from build123d import *

# Parameters (mm, degrees)
F0_W      = 50
F0_H      = 70
F1_DEPTH  = 67
F3_DEPTH  = 1.5
F4_W      = 29
F4_H      = 3.3
F5_DEPTH  = 67.001
F7_R      = 20
F8_DEPTH  = 1.5
F10_R     = 20
F11_DEPTH = 1.5
F12_R     = 3.15
F13_DEPTH = 12.5


with BuildPart() as f1:
    # F0 (on Front) → F1 (new body)
    with BuildSketch(Plane.XZ):
        with Locations((-25, 35)):
            Rectangle(F0_W, F0_H)
    extrude(amount=F1_DEPTH)

    # F2 (on face) → F3 (cut)
    with BuildSketch(Plane.YZ):
        Polygon((-67, 70), (-67, 65.2), (-38.1895705521, 35), (-33.5, 39.915755627), (-62.2, 70), align=None)
        Polygon((-33.5, 39.915755627), (-38.1895705521, 35), (-33.5, 30.084244373), (-28.8104294479, 35), align=None)
        Polygon((-67, 4.8), (-67, 0), (-62.2, 0), (-33.5, 30.084244373), (-38.1895705521, 35), align=None)
        Polygon((-4.8, 70), (-33.5, 39.915755627), (-28.8104294479, 35), (0, 65.2), (0, 70), align=None)
        Polygon((-33.5, 30.084244373), (-4.8, 0), (0, 0), (0, 4.8), (-28.8104294479, 35), align=None)
    extrude(amount=-F3_DEPTH, mode=Mode.SUBTRACT)

    # F4 (on face) → F5 (cut, through all)
    with BuildSketch(Plane(origin=(0, 0, 0), x_dir=(-1, 0, 0), z_dir=(0, 1, 0))):
        with Locations((35.5, 55.85)):
            Rectangle(F4_W, F4_H)
        with BuildLine():
            ThreePointArc((46, 27), (45.3525906995, 31.9175618569), (43.4544826719, 36.5))
            ThreePointArc((43.4544826719, 36.5), (8, 27), (43.4544826719, 17.5))
            ThreePointArc((43.4544826719, 17.5), (45.3525906995, 22.0824381431), (46, 27))
        make_face()
        with BuildLine():
            Line((50, 17.5), (50, 36.5))
            Line((50, 36.5), (43.4544826719, 36.5))
            ThreePointArc((43.4544826719, 36.5), (45.3525906995, 31.9175618569), (46, 27))
            ThreePointArc((46, 27), (45.3525906995, 22.0824381431), (43.4544826719, 17.5))
            Line((43.4544826719, 17.5), (50, 17.5))
        make_face()
    extrude(amount=-F5_DEPTH, mode=Mode.SUBTRACT)

    # F7 (on offset) → F8 (cut)
    with BuildSketch(Plane(origin=(0, -12.5, 0), x_dir=(-1, 0, 0), z_dir=(0, 1, 0))):
        with Locations((27, 27)):
            Circle(F7_R)
    extrude(amount=-F8_DEPTH, mode=Mode.SUBTRACT)

    # F10 (on offset) → F11 (cut)
    with BuildSketch(Plane(origin=(0, -56, 0), x_dir=(-1, 0, 0), z_dir=(0, 1, 0))):
        with Locations((27, 27)):
            Circle(F10_R)
    extrude(amount=-F11_DEPTH, mode=Mode.SUBTRACT)

    # F12 (on face) → F13 (cut, through all)
    with BuildSketch(Plane.XY.offset(70)):
        with Locations((-41.7, -33.5)):
            Circle(F12_R)
    extrude(amount=-F13_DEPTH, mode=Mode.SUBTRACT)


solid = f1.part
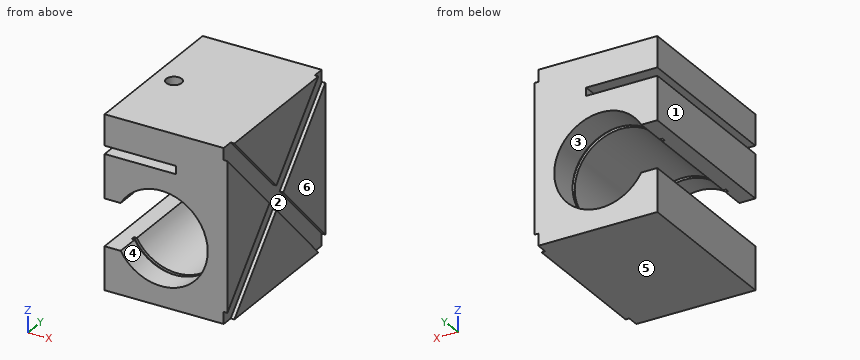
The listing builds one solid part. Answer for the finished solid, in the listing's coordinates (mm). Face numbers are marked on the shaded views. A direction names the side the tool comes from. Give positions to 0.01 mm unless a question says otherwise; leave off trailing zeros. Loops run counter-clockwise (first coordinate to the right, second up) from the corner with the lowest first, then second, coordinate; pieces in that order, holes last. Notation, with made-up numbers: (63, 88.5) - (121, 88.5) arc R23 ccw to (121, 105.5) - close; hole circle Ø11 at (-11.5, 28). An arc over 180 degrees is marked (long way). Write each question's results on one line, items separated by ' | '.
1. Consider probe 1 along Z at (x, y) = (-44.5, -20); probe 2 along Z at (x, y) = (-27, -13); probe 3 along Z at (x, y) = (-18, -54). Determine where each line is inside the solid, lowest interval first. Write a range as from..to.
Resolved:
probe 1: z = 0..17.5, 36.5..54.2, 57.5..70 | probe 2: z = 0..7, 47..54.2, 57.5..70 | probe 3: z = 0..10.27, 43.73..70
2. Find section A-A, the plane x = -27. Write down the section's boundary in (y, z), then the cut area to 3 significant figures.
Resolved:
outline: (-67, 0) - (0, 0) - (0, 8) - (-12.5, 8) - (-12.5, 7) - (-14, 7) - (-14, 8) - (-56, 8) - (-56, 7) - (-57.5, 7) - (-57.5, 8) - (-67, 8) - close; (-67, 46) - (-57.5, 46) - (-57.5, 47) - (-56, 47) - (-56, 46) - (-14, 46) - (-14, 47) - (-12.5, 47) - (-12.5, 46) - (0, 46) - (0, 54.2) - (-67, 54.2) - close; (-67, 57.5) - (0, 57.5) - (0, 70) - (-67, 70) - close | area: 1,920 mm^2
3. Find section D-D, the plane x = -41.7. Count the separate pieces of the cut face and the enclosed holes in it, then the cut area to 3 significant figures.
Resolved:
separate pieces: 4 | enclosed holes: 0 | area: 2,770 mm^2
4. For a pull along X with two mould halves and no side action, classify the marked faces 3, 4, 5 and 6 as +X half, -X half, draft (parallel to the pull), parting line (faces both ways), or undercut.
Resolved:
face 3: undercut | face 4: undercut | face 5: draft | face 6: +X half
5. Which of the six approach directions +Z, -Z, +X, -X, +Y, -Y give full straight-line access (tool end or side, diameter ignored) to the marked faces 1 and 2?
Resolved:
face 1: +Z, -Z, -X, +Y, -Y | face 2: +X
6. Find section C-C, the plane x = -17. Write down the section's boundary in (y, z).
Resolved:
outline: (-67, 0) - (0, 0) - (0, 10.84) - (-12.5, 10.84) - (-12.5, 9.68) - (-14, 9.68) - (-14, 10.84) - (-56, 10.84) - (-56, 9.68) - (-57.5, 9.68) - (-57.5, 10.84) - (-67, 10.84) - close; (-67, 43.16) - (-57.5, 43.16) - (-57.5, 44.32) - (-56, 44.32) - (-56, 43.16) - (-14, 43.16) - (-14, 44.32) - (-12.5, 44.32) - (-12.5, 43.16) - (0, 43.16) - (0, 70) - (-67, 70) - close
